Could you check a few things on this model? Use its own coordinates, in mm. A direction names the side the tool comes from. Coordinates: 2 decimals unless noted, no trailing zeros. Write each loop counter-clockwise with the first axis right and the second up, starting at its lowest first coordinate (ties: lowest second). Pieces come first, ordered by that corner, then holes.
```python
from build123d import *

# Parameters (mm, degrees)
SKETCH1_R                           = 10
SKETCH1_R_2                         = 4
BOSS_EXTRUDE1_DEPTH                 = 40
SKETCH4_W                           = 2.1
SKETCH4_H                           = 10
CUT_EXTRUDE1_START                  = 10
SKETCH5_W                           = 20
SKETCH5_H                           = 6
CUT_EXTRUDE1_DEPTH                  = 1
SKETCH7_W                           = 2.1
SKETCH7_H                           = 10
F_4_2_4_2_DIAMETER_HOLE1_AT_2_COUNT = 2
F_4_2_4_2_DIAMETER_HOLE1_AT_2_PITCH = 10
F_4_2_4_2_DIAMETER_HOLE1_AT_3_COUNT = 2
F_4_2_4_2_DIAMETER_HOLE1_AT_3_PITCH = 20
CUT_EXTRUDE3_START                  = -10
SKETCH8_W                           = 20
SKETCH8_H                           = 40
CUT_EXTRUDE3_DEPTH                  = 1


with BuildPart() as part:
    # Sketch1 → Boss-Extrude1 (new body)
    with BuildSketch(Plane.XY):
        Circle(SKETCH1_R)
        Circle(SKETCH1_R_2, mode=Mode.SUBTRACT)
    extrude(amount=BOSS_EXTRUDE1_DEPTH)

    # Sketch4 → Ø4.2 (4.2) Diameter Hole2 (revolve, cut)
    with BuildSketch(Plane(origin=(0, 0, 20), x_dir=(0, 0, -1), z_dir=(1, 0, 0))):
        with Locations((1.05, 5)):
            Rectangle(SKETCH4_W, SKETCH4_H)
    revolve(axis=Axis((0, -6.35, 20), (0, 1, 0)), mode=Mode.SUBTRACT)

    # Sketch5 → Cut-Extrude1 (cut)
    with BuildSketch(Plane(origin=(0, 0, 0), x_dir=(1, 0, 0), z_dir=(0, 1, 0)).offset(CUT_EXTRUDE1_START)):
        with Locations((0, -20)):
            Rectangle(SKETCH5_W, SKETCH5_H)
    extrude(amount=-CUT_EXTRUDE1_DEPTH, mode=Mode.SUBTRACT)

    # Sketch7 → Ø4.2 (4.2) Diameter Hole1 (revolve, cut)
    with BuildSketch(Plane(origin=(0, 0, 30), x_dir=(0, 0, 1), z_dir=(1, 0, 0))):
        with Locations((1.05, 5)):
            Rectangle(SKETCH7_W, SKETCH7_H)
    f_4_2_4_2_diameter_hole1 = revolve(axis=Axis((0, 6.35, 30), (0, -1, 0)), mode=Mode.SUBTRACT)

    # Ø4.2 (4.2) Diameter Hole1 at 2: Ø4.2 (4.2) Diameter Hole1 ×2
    with Locations(*[(0, 0, -i * F_4_2_4_2_DIAMETER_HOLE1_AT_2_PITCH) for i in range(1, F_4_2_4_2_DIAMETER_HOLE1_AT_2_COUNT)]):
        add(f_4_2_4_2_diameter_hole1, mode=Mode.SUBTRACT)

    # Ø4.2 (4.2) Diameter Hole1 at 3: Ø4.2 (4.2) Diameter Hole1 ×2
    with Locations(*[(0, 0, -i * F_4_2_4_2_DIAMETER_HOLE1_AT_3_PITCH) for i in range(1, F_4_2_4_2_DIAMETER_HOLE1_AT_3_COUNT)]):
        add(f_4_2_4_2_diameter_hole1, mode=Mode.SUBTRACT)

    # Sketch8 → Cut-Extrude3 (cut)
    with BuildSketch(Plane(origin=(0, 0, 0), x_dir=(1, 0, 0), z_dir=(0, 1, 0)).offset(CUT_EXTRUDE3_START)):
        with Locations((0, -20)):
            Rectangle(SKETCH8_W, SKETCH8_H)
    extrude(amount=CUT_EXTRUDE3_DEPTH, mode=Mode.SUBTRACT)


solid = part.part
```
Item 1: I want a section at B-B, the plane x = 0. List the corners of the cut face in (y, z) for me, then the cut area to 3 significant figures.
Item 2: Will these pins go through, and if not, where does the flat tip stop? pin 1 Ø4 at (x, z) = (0, 20) entering from -Y; pin 2 Ø4 at (y, z) = (-5, 10) entering from +X; pin 3 Ø3 at (y, z) = (8, 12.5) entering from -X; pin 4 Ø5 at (x, z) = (-3, 22) entering from +Y.
Item 3: Which directions (+Z, -Z, +X, -X, +Y, -Y) give clear straight access to the entire face, cutting with the end or side of a thin tool? Please do faces 4 (the flat face through (-0.1, 9.4, 17)), 5 (the cylindrical face through (-2.082, -6.241, 9.727)), 6 (the flat face through (-3, -9, 20)).
Item 4: If we mould it in two halves opening along Z, with no side actions, what happens to faces 1 (the cylindrical face through (-2.95, 2.7, 19.72)), 2 (the cylindrical face through (-2.082, -6.241, 19.727)), 3 (the flat face through (2, -4, 0))? For each: released by +Z, released by -Z, zero draft, split by the parting line, or undercut.
Item 5: I want a section at A-A, the plane z = 20. List the corners of the cut face in (x, y) for me.
Item 6: I want a section at C-C, the plane y = 2. List the corners of the cut face in (x, z) for me.
Item 7: I want a section at D-D, the plane x = 3. List the corners of the cut face in (y, z) for me.
Item 8: If I drill on line 1 along Z through (x, y) = (0, -7.3); line 2 along Z through (x, y) = (-1.5, -5.75); line 3 along X through (y, z) = (-5.7, 30), over which ranges is the centre line in solid material (lowest first)?
Taken from the geometry:
1. outline: (-9, 0) - (-4, 0) - (-4, 7.9) - (-9, 7.9) - close; (-9, 12.1) - (-4, 12.1) - (-4, 17.9) - (-9, 17.9) - close; (-9, 22.1) - (-4, 22.1) - (-4, 27.9) - (-9, 27.9) - close; (-9, 32.1) - (-4, 32.1) - (-4, 40) - (-9, 40) - close; (4, 0) - (10, 0) - (10, 17) - (9, 17) - (9, 17.9) - (4, 17.9) - close; (4, 22.1) - (9, 22.1) - (9, 23) - (10, 23) - (10, 40) - (4, 40) - close
1. area: 350 mm2
2. pin 1: passes through
2. pin 2: stops at x = 9.54
2. pin 3: stops at x = -7.6
2. pin 4: stops at y = 9.97
3. face 4: +X, -X, +Y
3. face 5: -Y
3. face 6: +Z, -Z, +X, -X, -Y
4. face 1: zero draft
4. face 2: undercut
4. face 3: released by -Z
5. outline: (-4.36, -9) - (-2.1, -9) - (-2.1, -3.4) arc R4 cw to (-2.1, 3.4) - (-2.1, 9) - (-4.36, 9) arc R10 ccw to start; (2.1, -9) - (4.36, -9) arc R10 ccw to (4.36, 9) - (2.1, 9) - (2.1, 3.4) arc R4 cw to (2.1, -3.4) - close
6. outline: (-9.8, 0) - (-3.46, 0) - (-3.46, 40) - (-9.8, 40) - close; (3.46, 0) - (9.8, 0) - (9.8, 40) - (3.46, 40) - close
7. outline: (-9, 0) - (-2.65, 0) - (-2.65, 40) - (-9, 40) - close; (2.65, 0) - (9.54, 0) - (9.54, 17) - (9, 17) - (9, 23) - (9.54, 23) - (9.54, 40) - (2.65, 40) - close
8. line 1: z = 0 to 7.9, 12.1 to 17.9, 22.1 to 27.9, 32.1 to 40
8. line 2: z = 0 to 8.53, 11.47 to 18.53, 21.47 to 28.53, 31.47 to 40
8. line 3: x = -8.22 to -2.1, 2.1 to 8.22
